Drawing for the job (mm, zero at the part's lowest x, y, z). A direction names the side the tool comes from. Round coordinates to 2 decimals unless told otherwise and drop trailing zeros. Order: outer loops, then holes, each group sorted by start corner. A loop starts at its lowest first (then second) coordinate and runs counter-clockwise, first axis right, second up. Notation, with made-up numbers: (34.5, 18) - (55.5, 18) arc R26 cw to (55.5, 46) - close; hole circle Ø11 at (17, 16). An arc over 180 degrees is marked (long way). Put each result on its own line as item: value. Start each with the question number.
Item 1: Which spindle directions (+Z, -Z, +X, -X, +Y, -Y) get a long thin tool onto all of the face, cutting with end or side? Do the marked faces 1, 2 and 3. Say none if no direction does.
Item 2: Pin check, flat tips, straight feed: pin 1 Ø5 at (x, y) = (34.5, 17.5) entering from -Z; pin 2 Ø3 at (x, y) = (30, 5) entering from +Z; pin 3 Ø22.5 at (x, z) = (20, 20) entering from +Y; pin 4 Ø5 at (x, y) = (35.5, 4) entering from +Z. Stop position of each tip, or through.
Item 3: Saw through at A-A on z = 20. List the corners of the cut face in (x, y).
Item 4: Saw through at D-D on x = 6.5. List the corners of the cut face in (y, z), plus the area to 3 significant figures.
Item 5: Saw through at C-C on y = 18. List the corners of the cut face in (x, z), plus the area to 3 significant figures.
Item 6: Probe probe 1 along Z at (x, y) = (20, 5.75); probe 2 along X at (y, z) = (12.75, 20). List the from-to ranges inside material, lowest first.
Item 7: Mould opens along X. For the marked faces 4, 5 and 6 say: pulls with the +X half, pulls with the -X half, needs draft (parallel to the pull), parting line crosses it, or undercut.
Item 8: Saw through at B-B on x = 20. List the corners of the cut face in (y, z), plus the area to 3 significant figures.
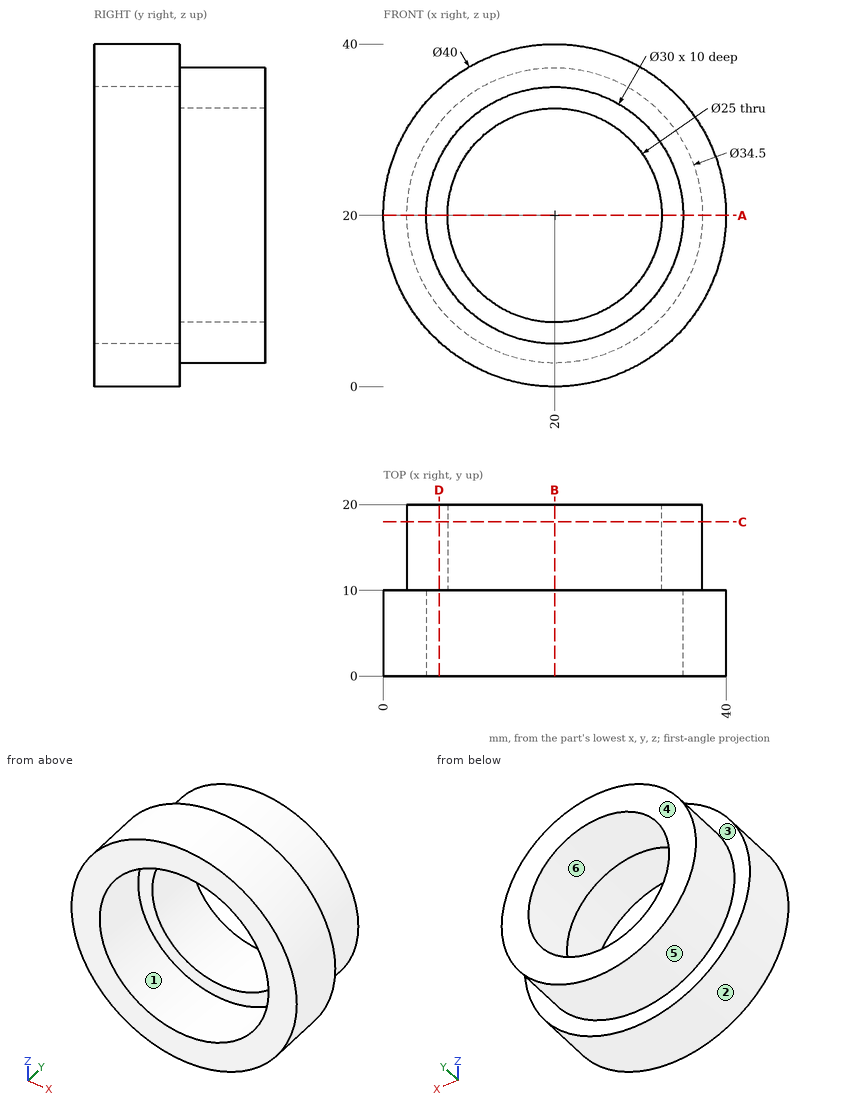
Results found:
1. face 1: -Y
1. face 2: +Y, -Y
1. face 3: +Y
2. pin 1: stops at z = 7.61
2. pin 2: stops at z = 38.1
2. pin 3: passes through
2. pin 4: stops at z = 35.2
3. outline: (0, 0) - (5, 0) - (5, 10) - (7.5, 10) - (7.5, 20) - (2.75, 20) - (2.75, 10) - (0, 10) - close; (32.5, 10) - (35, 10) - (35, 0) - (40, 0) - (40, 10) - (37.25, 10) - (37.25, 20) - (32.5, 20) - close
4. outline: (0, 5.24) - (10, 5.24) - (10, 9.26) - (20, 9.26) - (20, 30.74) - (10, 30.74) - (10, 34.76) - (0, 34.76) - (0, 26.54) - (10, 26.54) - (10, 13.46) - (0, 13.46) - close
4. area: 379 mm²
5. outline: circle Ø34.5 at (20, 20); hole circle Ø25 at (20, 20)
5. area: 444 mm²
6. probe 1: z = 0 to 5, 35 to 40
6. probe 2: x = 2.75 to 7.5, 32.5 to 37.25
7. face 4: needs draft
7. face 5: parting line crosses it
7. face 6: undercut
8. outline: (0, 0) - (10, 0) - (10, 2.75) - (20, 2.75) - (20, 7.5) - (10, 7.5) - (10, 5) - (0, 5) - close; (0, 35) - (10, 35) - (10, 32.5) - (20, 32.5) - (20, 37.25) - (10, 37.25) - (10, 40) - (0, 40) - close
8. area: 195 mm²
